```python
from build123d import *

# Parameters (mm, degrees)
SKETCH1_W           = 102
SKETCH1_H           = 69
SKETCH1_R           = 1.5
SKETCH1_W_2         = 82
SKETCH1_H_2         = 51.6
BOSS_EXTRUDE1_DEPTH = 2
SKETCH2_W           = 102
SKETCH2_H           = 69
SKETCH2_R           = 1.5
SKETCH2_W_2         = 82
SKETCH2_H_2         = 21.3
BOSS_EXTRUDE2_DEPTH = 2
FILLET1_R           = 3
SKETCH3_R           = 1.5
CUT_EXTRUDE1_DEPTH  = 62.605600395
SKETCH9_W           = 75.6
SKETCH9_H           = 6
BOSS_EXTRUDE5_DEPTH = 23.8
SKETCH10_R          = 1.5
CUT_EXTRUDE6_DEPTH  = 3
FILLET3_R           = 5
SKETCH11_W          = 14.6
SKETCH11_H          = 3
BOSS_EXTRUDE6_DEPTH = 18
SKETCH12_W          = 3
SKETCH12_H          = 53.8
BOSS_EXTRUDE7_DEPTH = 7.8
SKETCH13_W          = 3
SKETCH13_H          = 16.2
BOSS_EXTRUDE8_DEPTH = 3


with BuildPart() as part:
    # Sketch1 → Boss-Extrude1 (new body)
    with BuildSketch(Plane(origin=(0, 0, 0), x_dir=(1, 0, 0), z_dir=(0, 1, 0))):
        Rectangle(SKETCH1_W, SKETCH1_H)
        with Locations(Location((-48, 31.2, 0), (0, 0, 270))):
            Circle(SKETCH1_R, mode=Mode.SUBTRACT)
        with Locations(Location((40, 31.2, 0), (0, 0, 270))):
            Circle(SKETCH1_R, mode=Mode.SUBTRACT)
        with Locations(Location((40, -31.2, 0), (0, 0, 270))):
            Circle(SKETCH1_R, mode=Mode.SUBTRACT)
        with Locations(Location((-48, -31.2, 0), (0, 0, 270))):
            Circle(SKETCH1_R, mode=Mode.SUBTRACT)
        with Locations((-7, 0)):
            Rectangle(SKETCH1_W_2, SKETCH1_H_2, mode=Mode.SUBTRACT)
    extrude(amount=BOSS_EXTRUDE1_DEPTH)

    # Sketch2 → Boss-Extrude2 (add)
    with BuildSketch(Plane(origin=(0, 2, 0), x_dir=(1, 0, 0), z_dir=(0, 1, 0))):
        Rectangle(SKETCH2_W, SKETCH2_H)
        with Locations(Location((-44, 0, 0), (0, 0, 270))):
            Circle(SKETCH2_R, mode=Mode.SUBTRACT)
        with Locations(Location((30, 0, 0), (0, 0, 270))):
            Circle(SKETCH2_R, mode=Mode.SUBTRACT)
        with Locations((-7, 13.15)):
            Rectangle(SKETCH2_W_2, SKETCH2_H_2, mode=Mode.SUBTRACT)
        with Locations((-7, -13.15)):
            Rectangle(SKETCH2_W_2, SKETCH2_H_2, mode=Mode.SUBTRACT)
    extrude(amount=BOSS_EXTRUDE2_DEPTH)

    # Fillet1
    fillet1_edges = [part.edges().sort_by_distance(p)[0] for p in [
        (-48, 3, -2.5),
        (34, 3, -2.5),
        (34, 3, 2.5),
        (-48, 3, 2.5),
    ]]
    fillet(fillet1_edges, radius=FILLET1_R)

    # Sketch3 → Cut-Extrude1 (cut, through all)
    with BuildSketch(Plane.XZ.offset(-2)):
        with Locations(Location((-48, 31.2, 0), (0, 0, 270))):
            Circle(SKETCH3_R)
        with Locations(Location((-48, -31.2, 0), (0, 0, 270))):
            Circle(SKETCH3_R)
        with Locations(Location((40, -31.2, 0), (0, 0, 270))):
            Circle(SKETCH3_R)
        with Locations(Location((40, 31.2, 0), (0, 0, 270))):
            Circle(SKETCH3_R)
    extrude(amount=-CUT_EXTRUDE1_DEPTH, mode=Mode.SUBTRACT)

    # Sketch9 → Boss-Extrude5 (add)
    with BuildSketch(Plane(origin=(0, 4, 0), x_dir=(1, 0, 0), z_dir=(0, 1, 0))):
        with Locations((-4, 31.5)):
            Rectangle(SKETCH9_W, SKETCH9_H)
    extrude(amount=BOSS_EXTRUDE5_DEPTH)

    # Sketch10 → Cut-Extrude6 (cut)
    with BuildSketch(Plane.XY.offset(-28.5)):
        with BuildLine():
            Line((11, 27.8), (-19, 27.8))
            Line((-19, 27.8), (-19, 23))
            Line((-19, 23), (-15.5, 23))
            ThreePointArc((-15.5, 23), (-13.069617557, 21.085867885), (-14.360893582, 18.274592943))
            Line((-14.360893582, 18.274592943), (-19, 15.9))
            Line((-19, 15.9), (-19, 4))
            Line((-19, 4), (11, 4))
            Line((11, 4), (11, 15.9))
            Line((11, 15.9), (6.360893582, 18.274592943))
            ThreePointArc((6.360893582, 18.274592943), (5.069617557, 21.085867885), (7.5, 23))
            Line((7.5, 23), (11, 23))
            Line((11, 23), (11, 27.8))
        make_face()
        with Locations((-15.5, 20.5)):
            Circle(SKETCH10_R)
        with Locations((7.5, 20.5)):
            Circle(SKETCH10_R)
    extrude(amount=-CUT_EXTRUDE6_DEPTH, mode=Mode.SUBTRACT)

    # Fillet3
    # the kernel refuses this fillet: 5 mm, written as the material it adds along each edge
    with BuildSketch(Plane(origin=(-19, 15.9, -28.5), x_dir=(0, -1, 0), z_dir=(0, 0, -1))) as fillet3_piece_1:
        with BuildLine():
            CenterArc((FILLET3_R * 0.611525688318, -FILLET3_R), FILLET3_R, 90, 62.893714251)
            Line((-FILLET3_R * 0.278637134463, -FILLET3_R * 0.544357432916), (0, 0))
            Line((0, 0), (FILLET3_R * 0.611525688318, 0))
        make_face()
    extrude(amount=3)
    with BuildSketch(Plane(origin=(11, 15.9, -28.5), x_dir=(0, -1, 0), z_dir=(0, 0, -1))) as fillet3_piece_2:
        with BuildLine():
            CenterArc((FILLET3_R * 0.611525688318, FILLET3_R), FILLET3_R, 207.106285749, 62.893714251)
            Line((-FILLET3_R * 0.278637134463, FILLET3_R * 0.544357432916), (0, 0))
            Line((0, 0), (FILLET3_R * 0.611525688318, 0))
        make_face()
    extrude(amount=3)
    with BuildSketch(Plane(origin=(11, 23, -28.5), x_dir=(-0.9999202818433616, -0.012626557658055267, 0), z_dir=(0, 0, -1))) as fillet3_piece_3_section:
        with BuildLine():
            CenterArc((4.938381933, 4.911215506), FILLET3_R, 180.723467688, 78.463040967)
            Line((-0.061219476, 4.848082717), (-0.561179617, 4.841769438))
            Line((-0.561179617, 4.841769438), (-0.499960141, -0.006313279))
            Line((-0.499960141, -0.006313279), (0.006313279, -0.499960141))
            ThreePointArc((0.006313279, -0.499960141), (3.506034265, -0.455767189), (3.906512595, -0.491121551))
            Line((3.906512595, -0.491121551), (4.000318898, 0))
        make_face()
    fillet3_piece_3 = extrude(amount=3, mode=Mode.PRIVATE)
    fillet3_piece_3 = split(fillet3_piece_3, bisect_by=Plane(origin=(10.155931767, 27.8, -30), z_dir=(0, -1, 0)), keep=Keep.TOP, mode=Mode.PRIVATE)
    add(fillet3_piece_3)
    with BuildSketch(Plane(origin=(-19, 23, -28.5), x_dir=(0, 1, 0), z_dir=(0, 0, -1))) as fillet3_piece_4_section:
        with BuildLine():
            CenterArc((4.848469228, 5), FILLET3_R, 191.536959033, 78.463040967)
            Line((-0.050510257, 4), (-0.540408206, 3.9))
            ThreePointArc((-0.540408206, 3.9), (-0.5, 3.5), (-0.5, 0))
            Line((-0.5, 0), (0, -0.5))
            Line((0, -0.5), (4.848469228, -0.5))
            Line((4.848469228, -0.5), (4.848469228, 0))
        make_face()
    fillet3_piece_4 = extrude(amount=3, mode=Mode.PRIVATE)
    fillet3_piece_4 = split(fillet3_piece_4, bisect_by=Plane(origin=(-18.155931767, 27.8, -30), z_dir=(0, -1, 0)), keep=Keep.TOP, mode=Mode.PRIVATE)
    add(fillet3_piece_4)

    # Sketch11 → Boss-Extrude6 (add)
    with BuildSketch(Plane(origin=(0, 4, 0), x_dir=(1, 0, 0), z_dir=(0, 1, 0))):
        with Locations((27.5, -33)):
            Rectangle(SKETCH11_W, SKETCH11_H)
    extrude(amount=BOSS_EXTRUDE6_DEPTH)

    # Sketch12 → Boss-Extrude7 (add)
    with BuildSketch(Plane(origin=(0, 4, 0), x_dir=(1, 0, 0), z_dir=(0, 1, 0))):
        with Locations((-49.5, 1)):
            Rectangle(SKETCH12_W, SKETCH12_H)
    extrude(amount=BOSS_EXTRUDE7_DEPTH)

    # Sketch13 → Boss-Extrude8 (add)
    with BuildSketch(Plane(origin=(0, 11.8, 0), x_dir=(1, 0, 0), z_dir=(0, 1, 0))):
        with Locations((-49.5, -17.8)):
            Rectangle(SKETCH13_W, SKETCH13_H)
    extrude(amount=BOSS_EXTRUDE8_DEPTH)


solid = part.part
```
Here's how the part is built. I have some questions about the finished solid (model axes, mm). A direction names the side the tool comes from. Coordinates: 2 decimals unless noted, no trailing zeros. Loops run counter-clockwise (first coordinate to the right, second up) from the corner with the lowest first, then second, coordinate; pieces in that order, holes last. Notation, with made-up numbers: (53, -36.5) -> (85, -36.5) arc R36 ccw to (85, -1.5) -> close; hole circle Ø9 at (-32.5, -26). An arc over 180 degrees is marked (long way). Return JSON: item names as keys, results as strings.
1) If we section it at D-D, the plane z = -21: Write out the boundary of the cut face in (x, y), then the cut area to 3 significant figures.
Results below:
{"outline": "(-51, 0) -> (-48, 0) -> (-48, 11.8) -> (-51, 11.8) -> close; (34, 0) -> (51, 0) -> (51, 4) -> (34, 4) -> close", "area": "103 mm²"}
2) I need wall thicknesses on line 1 (X direction, y = 1, z = 31.2); line 2 (Z direction, x = 40, y = 1); line 3 (Z direction, x = 33, y = 12.5). Which ranges of each line are inside material? Lowest first, please. Write a range as from..to.
Results below:
{"line 1": "-51..-49.5, -46.5..38.5, 41.5..51", "line 2": "-34.5..-32.7, -29.7..29.7, 32.7..34.5", "line 3": "-34.5..-28.5, 31.5..34.5"}
3) Will these pins go through, and if not, where does the flat tip stop? pin 1 (3 mm diameter, centred on y = 6.5, z = -17.5, fed in from +X); pin 2 (2.5 mm diameter, centred on y = 10.5, z = -29.5, fed in from +X); pin 3 (1.8 mm diameter, centred on x = 7.5, y = 20.5, fed in from +Z); pin 4 (1 mm diameter, centred on x = -8.5, z = -3.5, fed in from +Y).
Results below:
{"pin 1": "x = -48", "pin 2": "x = 33.8", "pin 3": "z = -31.5", "pin 4": "through"}
4) For faces 5 (the face through (-17.8, 24.6, -30)), 6 (the face through (-50, 13, 9.7)), 7 (the face through (33.1, 3.01, 3.36)), 8 (the face through (10.25, 15.48, -29.98)), which set-ups out of +Z, -Z, +X, -X, +Y, -Y let a thin tool reach every point of the face, with its end or its side?
Results below:
{"face 5": "+Z, +Y", "face 6": "-Z, +X, -X, +Y", "face 7": "+Y, -Y", "face 8": "+Z"}
5) If we section it at A-A, the plane x = -5.5: Write out the boundary of the cut face in (y, z), then the cut area to 3 significant figures.
Results below:
{"outline": "(0, -34.5) -> (27.8, -34.5) -> (27.8, -31.5) -> (4, -31.5) -> (4, -23.8) -> (2, -23.8) -> (2, -25.8) -> (0, -25.8) -> close; (0, 25.8) -> (2, 25.8) -> (2, 23.8) -> (4, 23.8) -> (4, 34.5) -> (0, 34.5) -> close; (2, -2.5) -> (4, -2.5) -> (4, 2.5) -> (2, 2.5) -> close", "area": "159 mm²"}
6) If we section it at C-C, the plane z = 0: Write out the boundary of the cut face in (x, y), then the cut area to 3 significant figures.
Results below:
{"outline": "(-51, 0) -> (-48, 0) -> (-48, 2) -> (-45.5, 2) -> (-45.5, 4) -> (-48, 4) -> (-48, 11.8) -> (-51, 11.8) -> close; (-42.5, 2) -> (28.5, 2) -> (28.5, 4) -> (-42.5, 4) -> close; (31.5, 2) -> (34, 2) -> (34, 0) -> (51, 0) -> (51, 4) -> (31.5, 4) -> close", "area": "255 mm²"}
7) Thinking about a two-plate mould opening in Y: for faces 1 (the face through (-19, 8, -30)), 2 (the face through (27, 22, 33)), 3 (the face through (-8, 1, 25.8)), 4 (the face through (-18.286, 15.418, -29.979)), which applies, +Y half, -Y half, draft (parallel to the pull), parting line (faces both ways), or undercut?
Results below:
{"face 1": "undercut", "face 2": "+Y half", "face 3": "draft", "face 4": "undercut"}
8) If we section it at B-B, the plane y = 9.75: Write out the boundary of the cut face in (x, z).
Results below:
{"outline": "(-51, -27.9) -> (-48, -27.9) -> (-48, 25.9) -> (-51, 25.9) -> close; (-41.8, -34.5) -> (33.8, -34.5) -> (33.8, -28.5) -> (11, -28.5) -> (11, -31.5) -> (-19, -31.5) -> (-19, -28.5) -> (-41.8, -28.5) -> close; (20.2, 31.5) -> (34.8, 31.5) -> (34.8, 34.5) -> (20.2, 34.5) -> close"}
